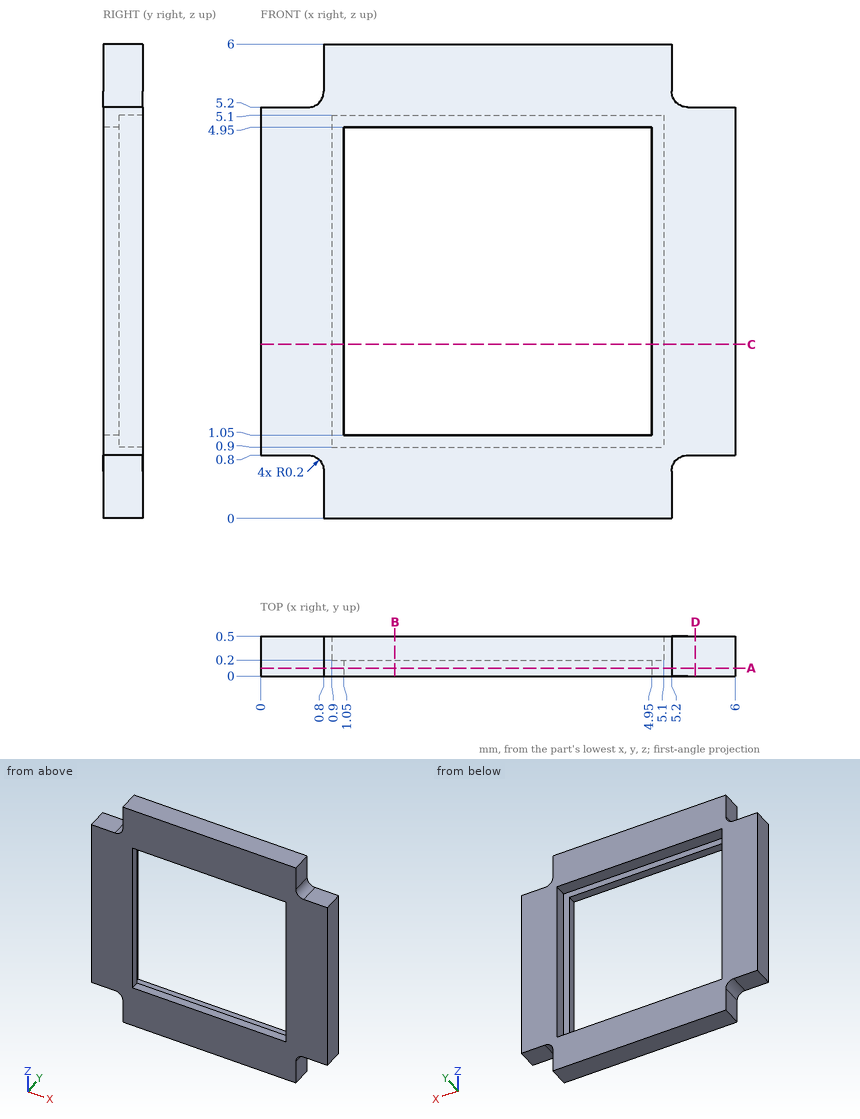
Geometry: see drawing. Coordinates: mm, zero at the bounding-box minimum. Give positions to 0.01 mm unless a question says otherwise; leave off trailing zeros. Loops run counter-clockwise (first coordinate to the right, second up) from the corner with the lowest first, then second, coordinate; pieces in that order, holes last. Notation, with made-up numbers: M -10.75,60 L 36.25,60 A14 cw 36.25,73 Z; hole C -15.5,10.5 d7. An arc over 180 degrees is marked long. Use one line per item in the form item = value.
1. Line query: L1, parallel to X at y = 0.45, z = 1.7; L2, parallel to X at y = 0.15, z = 1.65. Output: solid intervals per line, ascending.
Numbers:
L1 = 0 to 0.9, 5.1 to 6
L2 = 0 to 1.05, 4.95 to 6
2. Section query D-D, the plane x = 5.5. Return the cut outline in (y, z).
Numbers:
outline = M 0,0.8 L 0.5,0.8 L 0.5,5.2 L 0,5.2 Z
3. Section query B-B, the plane x = 1.7. Return the cut outline in (y, z).
Numbers:
outline = M 0,0 L 0.5,0 L 0.5,0.9 L 0.2,0.9 L 0.2,1.05 L 0,1.05 Z; M 0,4.95 L 0.2,4.95 L 0.2,5.1 L 0.5,5.1 L 0.5,6 L 0,6 Z
4. Section query C-C, the plane z = 2.2. Return the cut outline in (x, y).
Numbers:
outline = M 0,0 L 1.05,0 L 1.05,0.2 L 0.9,0.2 L 0.9,0.5 L 0,0.5 Z; M 4.95,0 L 6,0 L 6,0.5 L 5.1,0.5 L 5.1,0.2 L 4.95,0.2 Z
5. Section query A-A, the plane y = 0.1. Return the cut outline in (x, z), and give its area (3 significant figures).
Numbers:
outline = M 0,0.8 L 0.6,0.8 A0.2 cw 0.8,0.6 L 0.8,0 L 5.2,0 L 5.2,0.6 A0.2 cw 5.4,0.8 L 6,0.8 L 6,5.2 L 5.4,5.2 A0.2 cw 5.2,5.4 L 5.2,6 L 0.8,6 L 0.8,5.4 A0.2 cw 0.6,5.2 L 0,5.2 Z; hole M 1.05,1.05 L 4.95,1.05 L 4.95,4.95 L 1.05,4.95 Z
area = 18.3 mm²
